Autodesk Inventor part; units mm, degrees
ref_plane "YZ Plane" through (0, 0, 0) normal (1, 0, 0) x (0, 1, 0)
ref_plane "XZ Plane" through (0, 0, 0) normal (0, 1, 0) x (-1, 0, 0)
ref_plane "XY Plane" through (0, 0, 0) normal (0, 0, 1) x (1, 0, 0)
sketch "Esboço1" plane through (0, 0, 0) normal (0, 0, 1) x (1, 0, 0)
  line L0 (-50.5, -37) -> (50.5, -37)
  line L1 (50.5, -37) -> (50.5, 37)
  line L2 (50.5, 37) -> (-50.5, 37)
  line L3 (-50.5, 37) -> (-50.5, -37)
  point P0 (0, 0)
  point P1 (0, 0)
  dimension "d17" = 101
  dimension "d18" = 74
  dimension "d19" = 50.5
  dimension "d20" = 37
  dimension "d21" = 50.5
  dimension "d22" = 37
extrude "Extrusão1" add sketch "Esboço1" against normal blind 2
sketch "Esboço2" plane through (0, 0, 0) normal (0, 0, 1) x (1, 0, 0)
  line L0 (-50.5, -37) -> (-50.5, 37)
  line L1 (-50.5, 37) -> (50.5, 37)
  line L2 (-46.5, 37) -> (-46.5, -37) construction
  line L3 (50.5, -37) -> (-50.5, -37)
  line L4 (46.5, 37) -> (46.5, -37) construction
  line L5 (-50.5, 18.5) -> (50.5, 18.5) construction
  line L6 (-50.5, -18.5) -> (50.5, -18.5) construction
  line L7 (50.5, 37) -> (50.5, -37)
  point P0 (0, 0)
  point P1 (0, 0)
  point P2 (-46.5, 18.5)
  point P3 (-46.5, -18.5)
  point P4 (46.5, -18.5)
  point P5 (46.5, 18.5)
  dimension "d28" = 4
  dimension "d29" = 97
  dimension "d30" = 101
  dimension "d31" = 55.5
  dimension "d32" = 18.5
  dimension "d33" = 74
  dimension "d34" = 50.5
  dimension "d35" = 37
  dimension "d36" = 0
hole "Furo1" at (-46.5, 18.5, 0) at (-46.5, -18.5, 0) at (46.5, -18.5, 0) at (46.5, 18.5, 0) direction (0, 0, -1) diameter 2.459 end through all counterbore diameter 6.5 counterbore depth 1.5
sketch "Esboço3" plane through (0, 0, -2) normal (0, 0, -1) x (-1, 0, 0)
  line L0 (-36.25, 14.25) -> (-36.25, 21.4827)
  line L1 (-36.0982, 21.8416) -> (-33.0537, 24.7952)
  line L2 (-32.75, 25.5129) -> (-32.75, 29.7)
  line L3 (-32.25, 30.2) -> (-13.75, 30.2)
  line L4 (-10.25, 14.25) -> (-10.25, 21.4827)
  line L5 (-12.9463, 24.7952) -> (-9.9018, 21.8416)
  line L6 (-13.25, 29.7) -> (-13.25, 25.5129)
  line L7 (-27.134, 10.7) -> (-18.866, 10.7)
  line L8 (-13.8, 11.25) -> (-32.2, 11.25)
  line L9 (-13.8, 10.2) -> (-32.2, 10.2)
  arc A0 (-36.25, 14.25) -> (-32.2, 10.2) centre (-32.2, 14.25) ccw
  line L10 (-36.25, 14.25) -> (-36.25, 21.4827)
  arc A1 (-13.8, 10.2) -> (-9.75, 14.25) centre (-13.8, 14.25) ccw
  line L11 (-9.75, 21.4827) -> (-9.75, 14.25)
  line L12 (-12.9463, 24.7952) -> (-9.9018, 21.8416)
  line L13 (-32.25, 30.2) -> (-13.75, 30.2)
  line L14 (-13.25, 29.7) -> (-13.25, 25.5129)
  arc A2 (-13.25, 29.7) -> (-13.75, 30.2) centre (-13.75, 29.7) ccw
  arc A3 (-13.25, 25.5129) -> (-12.9463, 24.7952) centre (-12.25, 25.5129) ccw
  arc A4 (-9.75, 21.4827) -> (-9.9018, 21.8416) centre (-10.25, 21.4827) ccw
  arc A5 (-32.25, 30.2) -> (-32.75, 29.7) centre (-32.25, 29.7) ccw
  arc A6 (-36.0982, 21.8416) -> (-36.25, 21.4827) centre (-35.75, 21.4827) ccw
  arc A7 (-33.0537, 24.7952) -> (-32.75, 25.5129) centre (-33.75, 25.5129) ccw
  line L15 (-36.75, 9.7) -> (-9.25, 9.7)
  line L16 (-9.25, 9.7) -> (-9.25, 30.7)
  line L17 (-9.25, 30.7) -> (-36.75, 30.7)
  line L18 (-36.75, 9.7) -> (-36.75, 30.7)
  line L19 (9.75, 14.25) -> (9.75, 21.4827)
  arc A8 (9.75, 14.25) -> (13.8, 10.2) centre (13.8, 14.25) ccw
  line L20 (32.2, 10.2) -> (13.8, 10.2)
  arc A9 (32.903, 10.7703) -> (35.75, 14.25) centre (32.2, 14.25) ccw
  arc A10 (32.2, 10.2) -> (36.25, 14.25) centre (32.2, 14.25) ccw
  line L21 (36.25, 21.4827) -> (36.25, 14.25)
  line L22 (13.75, 30.2) -> (32.25, 30.2)
  line L23 (-36.25, -24.75) -> (-36.25, -17.5173)
  arc A11 (-36.25, -24.75) -> (-32.2, -28.8) centre (-32.2, -24.75) ccw
  line L24 (-13.8, -28.8) -> (-32.2, -28.8)
  arc A12 (-13.8, -28.8) -> (-9.75, -24.75) centre (-13.8, -24.75) ccw
  line L25 (-9.75, -17.5173) -> (-9.75, -24.75)
  line L26 (-32.25, -8.8) -> (-13.75, -8.8)
  line L27 (13.75, -8.8) -> (32.25, -8.8)
  line L28 (9.75, -24.75) -> (9.75, -17.5173)
  arc A13 (9.75, -24.75) -> (13.8, -28.8) centre (13.8, -24.75) ccw
  line L29 (32.2, -28.8) -> (13.8, -28.8)
  arc A14 (32.2, -28.8) -> (36.25, -24.75) centre (32.2, -24.75) ccw
  line L30 (36.25, -17.5173) -> (36.25, -24.75)
  line L31 (9.25, 30.7) -> (36.75, 30.7)
  line L32 (36.75, 30.7) -> (36.75, 9.7)
  line L33 (36.75, 9.7) -> (9.25, 9.7)
  line L34 (9.25, 9.7) -> (9.25, 30.7)
  line L35 (-36.75, -8.3) -> (-36.75, -29.3)
  line L36 (-36.75, -29.3) -> (-9.25, -29.3)
  line L37 (-9.25, -29.3) -> (-9.25, -8.3)
  line L38 (-9.25, -8.3) -> (-36.75, -8.3)
  line L39 (9.25, -8.3) -> (9.25, -29.3)
  line L40 (9.25, -29.3) -> (36.75, -29.3)
  line L41 (36.75, -29.3) -> (36.75, -8.3)
  line L42 (36.75, -8.3) -> (9.25, -8.3)
  point P0 (0, 0)
  dimension "d51" = 1
  dimension "d52" = 27
  dimension "d53" = 19.45
  dimension "d54" = 1.55
  dimension "d67" = 0.5
  dimension "d68" = 0.5
  dimension "d69" = 27
  dimension "d70" = 27
  dimension "d71" = 45.5
  dimension "d72" = 73
  dimension "d73" = 20.5
  dimension "d74" = 0.5
  dimension "d75" = 18.5
  dimension "d76" = 39.5
  dimension "d77" = 18.5
  dimension "d78" = 0.5
extrude "Extrusão3" cut sketch "Esboço3" against normal blind 10 contours L0 A6 L1 A7 L2 A5 L3 A2 L6 A3 L5 A4 L11 A1 L9 A0 | L18 L17 L16 L15 | L31 L32 L33 L34 | L38 L37 L36 L35 | L42 L41 L40 L39
properties part number "Ra-Manager_Painel-Placas_Tras_Plugs"
Can you work these out from the model? Positions are in its coordinate system, mm. A direction names the side the tool comes from. Coordinates: 2 decimals unless noted, no trailing zeros. Order: outer loops, then holes, each group sorted by start corner. A loop starts at its lowest first (then second) coordinate and runs counter-clockwise, first axis right, second up. Notation, with made-up numbers: (-40, 6) -> (6, 6) arc R35 ccw to (6, 44) -> close; hole circle Ø10 at (-24.5, 8). An arc over 180 degrees is marked (long way). Write each question's results on one line, items separated by ' | '.
Item 1: Which directions (+Z, -Z, +X, -X, +Y, -Y) give clear straight access to the entire face, cutting with the end or side of a thin tool? Please do faces 1 (the face through (1, 37, -1)), 2 (the face through (48.478, 21.079, -0.76)), 3 (the face through (9.25, -19, -1)).
Results are:
face 1: +Z, -Z, +X, -X, +Y | face 2: +Z | face 3: +Z, -Z
Item 2: If I drill on line 1 along Y through (x, z) = (32, -0.7); line 2 along Y through (x, z) = (46.5, -0.45); line 3 along X through (y, z) = (-18.5, -0.9), over which ranges is the centre line in solid material (lowest first)?
Results are:
line 1: -37 to -29.3, -8.3 to 9.7, 30.7 to 37 | line 2: -37 to -21.75, -15.25 to 15.25, 21.75 to 37 | line 3: -50.5 to -49.75, -43.25 to -36.75, -9.25 to 9.25, 36.75 to 43.25, 49.75 to 50.5
Item 3: I want a section at A-A, the plane x = 46.5. Write out the boundary of the cut face in (y, z), then the cut area to 3 significant figures.
Results are:
outline: (-37, -2) -> (-19.73, -2) -> (-19.73, -1.5) -> (-21.75, -1.5) -> (-21.75, 0) -> (-37, 0) -> close; (-17.27, -2) -> (17.27, -2) -> (17.27, -1.5) -> (15.25, -1.5) -> (15.25, 0) -> (-15.25, 0) -> (-15.25, -1.5) -> (-17.27, -1.5) -> close; (19.73, -2) -> (37, -2) -> (37, 0) -> (21.75, 0) -> (21.75, -1.5) -> (19.73, -1.5) -> close | area: 126 mm²
Item 4: I'm going to push a flat-ended pin straight in: pin 1 Ø2 at (x, y) = (-45, 18.5) entering from +Z. Where does the tip first touch, or does it pass through?
Results are:
pin 1: z = -1.5
Item 5: If we mould it in two halves opening along X, with no side actions, what happens to faces 4 (the face through (50.5, -1, -1)), 5 (the face through (-23, 9.7, -1)), 6 (the face through (-1, 1, 0))? For each: +X half, -X half, draft (parallel to the pull), parting line (faces both ways), or undercut.
Results are:
face 4: +X half | face 5: undercut | face 6: draft
Item 6: I want a section at C-C, the plane z = -0.7. Count the separate pieces of the cut face and the enclosed holes in it, then the cut area to 3 significant figures.
Results are:
separate pieces: 1 | enclosed holes: 8 | area: 5,030 mm²
Item 7: I want a section at D-D, the plane y = -18.5. Write out the boundary of the cut face in (x, z), then the cut area to 3 significant figures.
Results are:
outline: (-50.5, -2) -> (-47.73, -2) -> (-47.73, -1.5) -> (-49.75, -1.5) -> (-49.75, 0) -> (-50.5, 0) -> close; (-45.27, -2) -> (-36.75, -2) -> (-36.75, 0) -> (-43.25, 0) -> (-43.25, -1.5) -> (-45.27, -1.5) -> close; (-9.25, -2) -> (9.25, -2) -> (9.25, 0) -> (-9.25, 0) -> close; (36.75, -2) -> (45.27, -2) -> (45.27, -1.5) -> (43.25, -1.5) -> (43.25, 0) -> (36.75, 0) -> close; (47.73, -2) -> (50.5, -2) -> (50.5, 0) -> (49.75, 0) -> (49.75, -1.5) -> (47.73, -1.5) -> close | area: 70.0 mm²
Item 8: I want a section at B-B, the plane y = -26. Write out the boundary of the cut face in (x, z).
Results are:
outline: (-50.5, -2) -> (-36.75, -2) -> (-36.75, 0) -> (-50.5, 0) -> close; (-9.25, -2) -> (9.25, -2) -> (9.25, 0) -> (-9.25, 0) -> close; (36.75, -2) -> (50.5, -2) -> (50.5, 0) -> (36.75, 0) -> close
